Could you check a few things on this model? Use its own coordinates, in mm. A direction names the side the tool comes from. Coordinates: 2 decimals unless noted, no trailing zeros. Loops run counter-clockwise (first coordinate to the right, second up) from the corner with the lowest first, then second, coordinate; pieces in that order, holes last. Notation, with made-up numbers: M -15.5,-8.5 L 21.5,-8.5 A20 ccw 21.5,12.5 Z; hole C -9.75,-23 d8. An arc over 180 degrees is marked long. Write each question's results on one line, items separated by ' | '.
```python
from build123d import *

# Parameters (mm, degrees)
SKETCH1_R           = 42.5
BOSS_EXTRUDE1_DEPTH = 200
SKETCH2_R           = 35
BOSS_EXTRUDE2_DEPTH = 110
FILLET1_R           = 10
SKETCH3_R           = 10
CUT_EXTRUDE1_DEPTH  = 40
FILLET2_R           = 10


with BuildPart() as part:
    # Sketch1 → Boss-Extrude1 (new body)
    with BuildSketch(Plane(origin=(0, 0, 0), x_dir=(1, 0, 0), z_dir=(0, 1, 0))):
        Circle(SKETCH1_R)
    extrude(amount=BOSS_EXTRUDE1_DEPTH)

    # Sketch2 → Boss-Extrude2 (add)
    with BuildSketch(Plane(origin=(0, 0, 0), x_dir=(0, 0, -1), z_dir=(1, 0, 0))):
        with Locations((0, 155)):
            Circle(SKETCH2_R)
    extrude(amount=BOSS_EXTRUDE2_DEPTH)

    # Fillet1
    fillet1_edges = [part.edges().sort_by_distance(p)[0] for p in [
        (-42.5, 200, 0),
    ]]
    fillet(fillet1_edges, radius=FILLET1_R)

    # Sketch3 → Cut-Extrude1 (cut)
    with BuildSketch(Plane(origin=(110, 0, 0), x_dir=(0, 0, -1), z_dir=(1, 0, 0))):
        with Locations((0, 155)):
            Circle(SKETCH3_R)
    extrude(amount=-CUT_EXTRUDE1_DEPTH, mode=Mode.SUBTRACT)

    # Fillet2
    fillet2_edges = [part.edges().sort_by_distance(p)[0] for p in [
        (110, 155, 35),
    ]]
    fillet(fillet2_edges, radius=FILLET2_R)


solid = part.part
```
(1) Which directions (+Z, -Z, +X, -X, +Y, -Y) give clear straight access to the entire face, cutting with the end or side of a thin tool? Please do faces 4 (the flat face through (-1, 0, -1)), 5 (the flat face through (70, 155, 0)).
Reported:
face 4: +Z, -Z, +X, -X, -Y | face 5: +X
(2) Imagine slicing it at A-A, the plane y = 155. List the corners of the cut face in (x, z) for me.
Reported:
outline: M 24.11,-35 L 100,-35 A10 ccw 110,-25 L 110,-10 L 70,-10 L 70,10 L 110,10 L 110,25 A10 ccw 100,35 L 24.11,35 A42.5 ccw long Z
(3) Will these pins go through, and if not, where does the flat tip stop? P1, Ø4, axis at y = 131, z = 32.5, coming from the +X side; P2, Ø4, axis at y = 58, z = -17.5, coming from the +X side; P3, Ø12, axis at x = 27, z = 31, coming from the +Y side.
Reported:
P1: stops at x = 29.6 | P2: stops at x = 39.57 | P3: stops at y = 199.65
(4) Imagine slicing it at B-B, the plane y = 30. List the corners of the cut face in (x, z) for me.
Reported:
outline: C 0,0 d85
(5) If we mould it in two halves opening along Z, with no side actions, what happens to faces 1 (the cylindrical face through (69.96, 141.59, -32.33)), 2 (the cylindrical face through (90.28, 145.24, 2.17)), 3 (the flat face through (110, 155, -11))? For each: released by +Z, released by -Z, zero draft, split by the parting line, or undercut.
Reported:
face 1: split by the parting line | face 2: undercut | face 3: zero draft
(6) Please list where these lines run through material, in increasing order: probe 1 along Y at (x, z) = (83.5, 0); probe 2 along Y at (x, z) = (78.5, -6); probe 3 along X at (y, z) = (151, 4). Write a range as from..to.
Reported:
probe 1: y = 120..145, 165..190 | probe 2: y = 120.52..147, 163..189.48 | probe 3: x = -42.31..70
